Input: part model. Units: mm. Frame: model coordinates. Face numbers are marked on the shaded views. A direction names the side the tool comes from. Coordinates: 2 decimals unless noted, no trailing zeros. Write each loop counter-clockwise with the first axis right and the second up, starting at its lowest first coordinate (ties: lowest second). Pieces come first, ordered by that corner, then holes. Notation, with made-up numbers: M 50.5,45.5 L 80.5,45.5 A24 ccw 80.5,57.5 Z; hole C 35,59.5 d8. An arc over 180 degrees is marked long. Write each question's results on one line, items separated by ' | '. Start each with the question number.
1. Section query C-C, the plane z = 33.25. Output: boundary loops of the cut face in (x, y).
2. Pull-direction query (X, two-part tool) for the marked faces 1, 2, 3 and 4; classes: +X half, -X half, draft (parallel to the pull), parting line (faces both ways), or undercut.
3. Ray query, probe 1 along Z at (x, y) = (33.5, 7.75); probe 2 along X at (y, z) = (1.55, 33.25); probe 3 along Z at (x, y) = (21, 1.25). Return the intervals inside material, ascending.
4. Set-up query: the marked faces 5, 6 and 7. Return all of +Z, -Z, +X, -X, +Y, -Y with unobstructed straight access to the full face (end or side cutting, diameter ignored); none if empty.
5. Section query A-A, the plane x = 20. Output: boundary loops of the cut face in (y, z), and give its area (3 significant figures).
6. First-contact query: pin 1 (5 mm diameter, centred on x = 0, z = -20, fed in from +Y). Flat tip, straight axial feed; report the tip coordinate or a pass-through.
7. Section query B-B, the plane z = 19. Output: boundary loops of the cut face in (x, y), and give its area (3 significant figures).
```python
from build123d import *

# Parameters (mm, degrees)
SKETCH1_R           = 2
SKETCH1_W           = 75
SKETCH1_H           = 24
BOSS_EXTRUDE1_DEPTH = 5
SKETCH2_W           = 75
SKETCH2_H           = 24
BOSS_EXTRUDE3_DEPTH = 3
SKETCH3_R           = 2
CUT_EXTRUDE1_DEPTH  = 5
FILLET2_R           = 5
SKETCH4_R           = 2
CUT_EXTRUDE2_DEPTH  = 5
SKETCH5_R           = 4
CUT_EXTRUDE3_DEPTH  = 2


with BuildPart() as part:
    # Sketch1 → Boss-Extrude1 (new body)
    with BuildSketch(Plane(origin=(0, 0, 0), x_dir=(1, 0, 0), z_dir=(0, 1, 0))):
        Polygon((8, -48), (83, -48), (99, -48), (99, 25), (83, 25), (83, 8), (8, 8), (8, 25), (-8, 25), (-8, -48), align=None)
        with Locations(Location((0, 0, 0), (0, 0, 270))):
            Circle(SKETCH1_R, mode=Mode.SUBTRACT)
        with Locations(Location((91, 0, 0), (0, 0, 270))):
            Circle(SKETCH1_R, mode=Mode.SUBTRACT)
        with Locations(Location((0, -13, 0), (0, 0, 270))):
            Circle(SKETCH1_R, mode=Mode.SUBTRACT)
        with Locations(Location((91, -13, 0), (0, 0, 270))):
            Circle(SKETCH1_R, mode=Mode.SUBTRACT)
        with Locations((45.5, -20)):
            Rectangle(SKETCH1_W, SKETCH1_H, mode=Mode.SUBTRACT)
    extrude(amount=BOSS_EXTRUDE1_DEPTH)

    # Sketch2 → Boss-Extrude3 (add)
    # profile 1 of 3: a face of its own
    with BuildSketch(Plane(origin=(0, 5, 0), x_dir=(1, 0, 0), z_dir=(0, 1, 0))):
        Polygon((-8, 25), (-8, -48), (96, -48), (99, -48), (99, 25), (96, 25), (96, -45), (-5, -45), (-5, 25), align=None)
    # profile 2 of 3: a face of its own
    with BuildSketch(Plane(origin=(0, 5, 0), x_dir=(1, 0, 0), z_dir=(0, 1, 0))):
        Polygon((8, 25), (5, 25), (5, 8), (5, 5), (86, 5), (86, 25), (83, 25), (83, 8), (8, 8), align=None)
    # profile 3 of 3: a face of its own
    with BuildSketch(Plane(origin=(0, 5, 0), x_dir=(1, 0, 0), z_dir=(0, 1, 0))):
        Polygon((86, -5), (86, -32), (86, -35), (5, -35), (5, -5), (83, -5), align=None)
        with Locations((45.5, -20)):
            Rectangle(SKETCH2_W, SKETCH2_H, mode=Mode.SUBTRACT)
    extrude(amount=BOSS_EXTRUDE3_DEPTH)

    # Sketch3 → Cut-Extrude1 (cut)
    with BuildSketch(Plane(origin=(0, 5, 0), x_dir=(1, 0, 0), z_dir=(0, 1, 0))):
        with Locations(Location((0, -40, 0), (0, 0, 270))):
            Circle(SKETCH3_R)
        with Locations(Location((91, -40, 0), (0, 0, 270))):
            Circle(SKETCH3_R)
        with Locations(Location((91, -26.5, 0), (0, 0, 270))):
            Circle(SKETCH3_R)
        with Locations(Location((0, -26.5, 0), (0, 0, 270))):
            Circle(SKETCH3_R)
        with Locations(Location((0, 12.5, 0), (0, 0, 270))):
            Circle(SKETCH3_R)
        with Locations(Location((91, 12.5, 0), (0, 0, 270))):
            Circle(SKETCH3_R)
        with Locations(Location((0, 20, 0), (0, 0, 270))):
            Circle(SKETCH3_R)
        with Locations(Location((91, 20, 0), (0, 0, 270))):
            Circle(SKETCH3_R)
        with Locations(Location((0, -33.25, 0), (0, 0, 270))):
            Circle(SKETCH3_R)
        with Locations(Location((91, -33.25, 0), (0, 0, 270))):
            Circle(SKETCH3_R)
        with Locations(Location((75.5, 0, 0), (0, 0, 270))):
            Circle(SKETCH3_R)
        with Locations(Location((65.5, 0, 0), (0, 0, 270))):
            Circle(SKETCH3_R)
        with Locations(Location((55.5, 0, 0), (0, 0, 270))):
            Circle(SKETCH3_R)
        with Locations(Location((45.5, 0, 0), (0, 0, 270))):
            Circle(SKETCH3_R)
        with Locations(Location((35.5, 0, 0), (0, 0, 270))):
            Circle(SKETCH3_R)
        with Locations(Location((25.5, 0, 0), (0, 0, 270))):
            Circle(SKETCH3_R)
        with Locations(Location((15.5, 0, 0), (0, 0, 270))):
            Circle(SKETCH3_R)
        with Locations(Location((55.5, -40, 0), (0, 0, 270))):
            Circle(SKETCH3_R)
        with Locations(Location((45.5, -40, 0), (0, 0, 270))):
            Circle(SKETCH3_R)
        with Locations(Location((15.5, -40, 0), (0, 0, 270))):
            Circle(SKETCH3_R)
        with Locations(Location((75.5, -40, 0), (0, 0, 270))):
            Circle(SKETCH3_R)
        with Locations(Location((65.5, -40, 0), (0, 0, 270))):
            Circle(SKETCH3_R)
        with Locations(Location((25.5, -40, 0), (0, 0, 270))):
            Circle(SKETCH3_R)
        with Locations(Location((35.5, -40, 0), (0, 0, 270))):
            Circle(SKETCH3_R)
    extrude(amount=-CUT_EXTRUDE1_DEPTH, mode=Mode.SUBTRACT)

    # Fillet2
    fillet2_edges = [part.edges().sort_by_distance(p)[0] for p in [
        (5, 6.5, 5),
        (5, 6.5, 35),
        (86, 6.5, 35),
        (86, 6.5, 5),
        (8, 4, -8),
        (83, 4, -8),
        (99, 4, 48),
        (-8, 4, 48),
        (8, 4, 8),
        (8, 4, 32),
        (83, 4, 32),
        (83, 4, 8),
        (96, 6.5, 45),
        (-5, 6.5, 45),
        (5, 6.5, -5),
        (86, 6.5, -5),
    ]]
    fillet(fillet2_edges, radius=FILLET2_R)

    # Sketch4 → Cut-Extrude2 (cut)
    with BuildSketch(Plane(origin=(0, 5, 0), x_dir=(1, 0, 0), z_dir=(0, 1, 0))):
        with Locations(Location((7.75, -40, 0), (0, 0, 270))):
            Circle(SKETCH4_R)
        with Locations(Location((83.25, -40, 0), (0, 0, 270))):
            Circle(SKETCH4_R)
    extrude(amount=-CUT_EXTRUDE2_DEPTH, mode=Mode.SUBTRACT)

    # Sketch5 → Cut-Extrude3 (cut)
    with BuildSketch(Plane.XZ):
        with Locations(Location((91, 0, 0), (0, 0, 270))):
            Circle(SKETCH5_R)
        with Locations(Location((91, 13, 0), (0, 0, 270))):
            Circle(SKETCH5_R)
        with Locations(Location((0, 0, 0), (0, 0, 270))):
            Circle(SKETCH5_R)
        with Locations(Location((0, 13, 0), (0, 0, 270))):
            Circle(SKETCH5_R)
    extrude(amount=-CUT_EXTRUDE3_DEPTH, mode=Mode.SUBTRACT)


solid = part.part
```
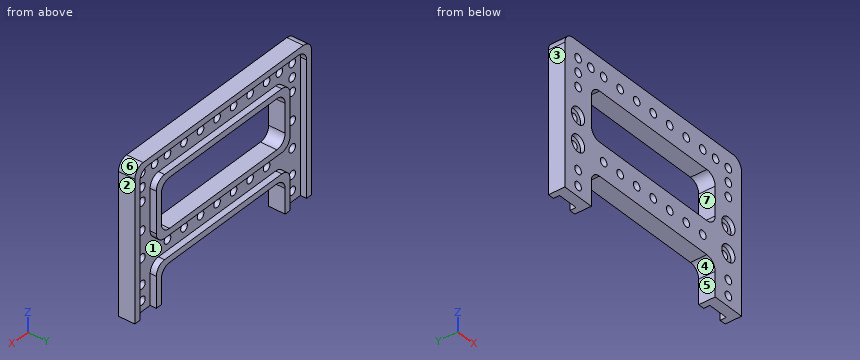
Answer:
1) outline: M -8,0 L -2,0 L -2,5 L -5,5 L -5,8 L -8,8 Z; M 2,0 L 89,0 L 89,5 L 84.8,5 L 84.8,8 L 6.2,8 L 6.2,5 L 2,5 Z; M 93,0 L 99,0 L 99,8 L 96,8 L 96,5 L 93,5 Z
2) face 1: undercut | face 2: +X half | face 3: -X half | face 4: undercut
3) probe 1: -8 to -5, 5 to 8, 32 to 35, 45 to 48 | probe 2: -8 to -2, 2 to 89, 93 to 99 | probe 3: -8 to 8, 32 to 48
4) face 5: -Z, +Y, -Y | face 6: +Z, +X, +Y, -Y | face 7: +Y, -Y
5) outline: M 0,-8 L 8,-8 L 8,-5 L 5,-5 L 5,5 L 8,5 L 8,8 L 0,8 Z; M 0,32 L 8,32 L 8,35 L 5,35 L 5,45 L 8,45 L 8,48 L 0,48 Z | area: 196 mm^2
6) pin 1: y = 5
7) outline: M -8,0 L 8,0 L 8,8 L 5,8 L 5,5 L -5,5 L -5,8 L -8,8 Z; M 83,0 L 99,0 L 99,8 L 96,8 L 96,5 L 86,5 L 86,8 L 83,8 Z | area: 196 mm^2
